```python
from build123d import *

# Parameters (mm, degrees)
SKETCH1_W           = 30
SKETCH1_H           = 23
BOSS_EXTRUDE1_DEPTH = 2
SKETCH3_R           = 1.5
SKETCH3_W           = 22
SKETCH3_H           = 10
CUT_EXTRUDE2_DEPTH  = 3


with BuildPart() as part:
    # Sketch1 → Boss-Extrude1 (new body)
    with BuildSketch(Plane(origin=(0, 0, 0), x_dir=(1, 0, 0), z_dir=(0, 1, 0))):
        Rectangle(SKETCH1_W, SKETCH1_H)
    extrude(amount=BOSS_EXTRUDE1_DEPTH)

    # Sketch3 → Cut-Extrude2 (cut)
    with BuildSketch(Plane(origin=(0, 2, 0), x_dir=(1, 0, 0), z_dir=(0, 1, 0))):
        with Locations(Location((-6.73, -8.5, 0), (0, 0, 270))):
            Circle(SKETCH3_R)
        with Locations(Location((9, -8.5, 0), (0, 0, 270))):
            Circle(SKETCH3_R)
        with Locations((1, 4.5)):
            Rectangle(SKETCH3_W, SKETCH3_H)
    extrude(amount=-CUT_EXTRUDE2_DEPTH, mode=Mode.SUBTRACT)


solid = part.part
```
Input: part model. Units: mm. Frame: model coordinates. A direction names the side the tool comes from. Coordinates: 2 decimals unless noted, no trailing zeros. Write each loop counter-clockwise with the first axis right and the second up, starting at its lowest first coordinate (ties: lowest second). Pieces come first, ordered by that corner, then holes. Notation, with made-up numbers: M -3.75,69.5 L 22.25,69.5 A26 ccw 22.25,99.5 Z; hole C 71.5,-38 d7. An arc over 180 degrees is marked long. Use one line per item in the form item = value.
Q1. Section A-A (z = 8.5). Return loops of the section in (x, y), plus the area to 3 significant figures.
Answer below:
outline = M -15,0 L -8.23,0 L -8.23,2 L -15,2 Z; M -5.23,0 L 7.5,0 L 7.5,2 L -5.23,2 Z; M 10.5,0 L 15,0 L 15,2 L 10.5,2 Z
area = 48.0 mm²
Q2. Section B-B (x = -6.73). Return loops of the section in (y, z), plus the area to 3 significant figures.
Answer below:
outline = M 0,-11.5 L 2,-11.5 L 2,-9.5 L 0,-9.5 Z; M 0,0.5 L 2,0.5 L 2,7 L 0,7 Z; M 0,10 L 2,10 L 2,11.5 L 0,11.5 Z
area = 20.0 mm²
Q3. Set-up query: faces 1 (the face through (0, 0, 2)), 2 (the face through (12, 1, -4)). Return all of +Z, -Z, +X, -X, +Y, -Y with unobstructed straight access to the full face (end or side cutting, diameter ignored); none if empty.
Answer below:
face_1 = +Z, -Z, +X, -X, -Y
face_2 = +Y, -Y
Q4. Material intervals for probe 1 along X at (y, z) = (0.45, 8.5); probe 2 along X at (y, z) = (1.6, -6.5); probe 3 along X at (y, z) = (1.15, 9.5), sorted ascending. Write a range as from..to.
Answer below:
probe_1 = -15..-8.23, -5.23..7.5, 10.5..15
probe_2 = -15..-10, 12..15
probe_3 = -15..-7.85, -5.61..7.88, 10.12..15
Q5. Section C-C (z = -5). Return loops of the section in (x, y).
Answer below:
outline = M -15,0 L -10,0 L -10,2 L -15,2 Z; M 12,0 L 15,0 L 15,2 L 12,2 Z
Q6. Draft query along Z for faces 3 (the face through (7.536, 1.014, 8.175)), 4 (the face through (0, 1, 11.5)), 5 (the face through (-15, 1, 0)). Return one class per face: released by +Z, released by -Z, zero draft, split by the parting line, or undercut.
Answer below:
face_3 = undercut
face_4 = released by +Z
face_5 = zero draft
Q7. Section D-D (y = 0.3). Return loops of the section in (x, z).
Answer below:
outline = M -15,-11.5 L 15,-11.5 L 15,11.5 L -15,11.5 Z; hole M -10,-9.5 L 12,-9.5 L 12,0.5 L -10,0.5 Z; hole C -6.73,8.5 d3; hole C 9,8.5 d3
